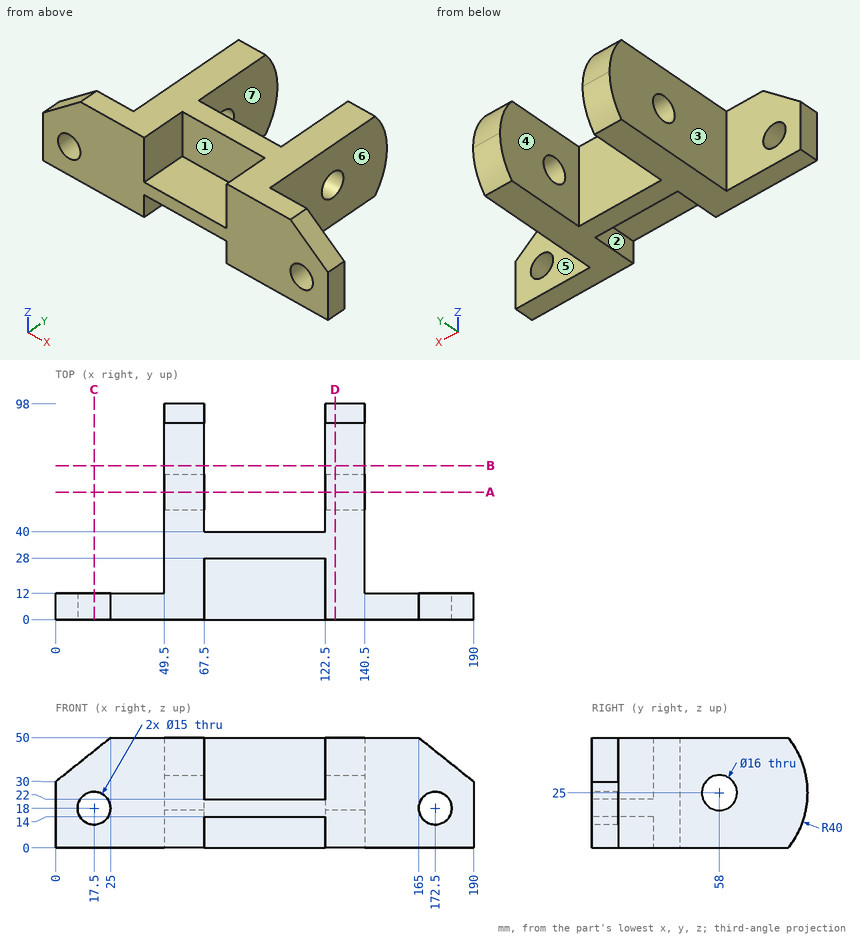
Geometry check sheet. Reference: drawing and pictorial views, mm from the part's lowest x, y, z. A direction names the side the tool comes from. Coordinates: 2 decimals unless noted, no trailing zeros. Order: outer loops, then holes, each group sorted by start corner. A loop starts at its lowest first (then second) coordinate and runs counter-clockwise, first axis right, second up. Notation, with made-up numbers: M -20,39 L 27,39 A8 cw 27,44 Z; hole C 7,50.5 d6. An arc over 180 degrees is marked long. Return JSON: item names as keys, results as strings.
1) Release check for a two-part mould opening along X. For the marked faces 5, 6 and 7 record: +X half, -X half, draft (parallel to the pull), parting line (faces both ways), or undercut.
Answer list:
{"face 5": "draft", "face 6": "+X half", "face 7": "undercut"}
2) Cross-section at D-D, the plane x = 127. Record the boundary of the cut face in (y, z), and give its area (3 significant figures).
Answer list:
{"outline": "M 0,0 L 89.22,0 A40 ccw 89.22,50 L 0,50 Z; hole C 58,25 d16", "area": "4,560 mm2"}
3) Cross-section at A-A, the plane y = 58. Record the boundary of the cut face in (x, z).
Answer list:
{"outline": "M 49.5,0 L 67.5,0 L 67.5,17 L 49.5,17 Z; M 49.5,33 L 67.5,33 L 67.5,50 L 49.5,50 Z; M 122.5,0 L 140.5,0 L 140.5,17 L 122.5,17 Z; M 122.5,33 L 140.5,33 L 140.5,50 L 122.5,50 Z"}
4) Cross-section at B-B, the plane y = 70. Record the boundary of the cut face in (x, z).
Answer list:
{"outline": "M 49.5,0 L 67.5,0 L 67.5,50 L 49.5,50 Z; M 122.5,0 L 140.5,0 L 140.5,50 L 122.5,50 Z"}
5) Access from +Z, -Z, +X, -X, +Y, -Y to the whole of each face (thin tool, end or side, straight path). Record for the marked faces 1, 2, 3 and 4.
Answer list:
{"face 1": "+Z, -Y", "face 2": "-Z, -Y", "face 3": "+Z, -Z, -X, +Y", "face 4": "+Z, -Z, +Y"}
6) Gauge pin test, flat ends, axial feed: pin 1 (13.5 mm diameter, centred on x = 17.5, z = 18, fed in from +Y); pin 2 (12 mm diameter, centred on x = 130, z = 13, fed in from -Y); pin 3 (11 mm diameter, centred on x = 98.5, z = 5.5, fed in from -Y); pin 4 (25 mm diameter, centred on y = 60, z = 22, fed in from +X). Record the tip position at first contact, or that the pin passes through.
Answer list:
{"pin 1": "through", "pin 2": "y = 0", "pin 3": "y = 28", "pin 4": "x = 140.5"}
7) Thickness scan on L1, parallel to X at y = 23, z = 41.5; L2, parallel to Y at x = 128, z = 25; L3, parallel to Y at x = 157, z = 19. Record the ranges inside material, lowest first. Write a range as [from, to].
Answer list:
{"L1": "[49.5, 67.5], [122.5, 140.5]", "L2": "[0, 50], [66, 98]", "L3": "[0, 12]"}
8) Cross-section at C-C, the plane x = 17.5. Record the boundary of the cut face in (y, z).
Answer list:
{"outline": "M 0,0 L 12,0 L 12,10.5 L 0,10.5 Z; M 0,25.5 L 12,25.5 L 12,44 L 0,44 Z"}
